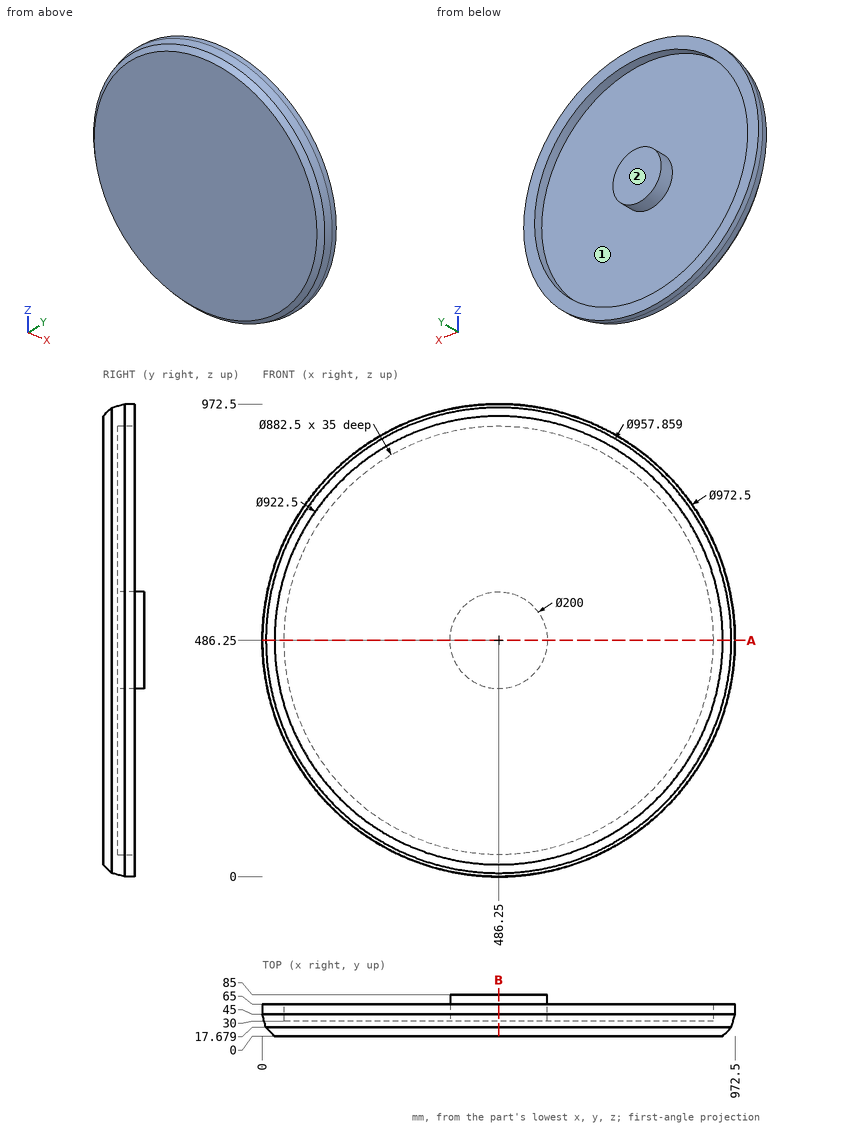
The figure shows three views and two pictorial views of one solid part (mm, origin at its lowest corner). Answer the questions. Give positions to 0.01 mm unless a question says otherwise; leave off trailing zeros. Order: outer loops, then holes, each group sorted by start corner. A loop starts at its lowest first (then second) coordinate and runs counter-clockwise, first axis right, second up. Notation, with made-up numbers: (50, 45.5) -> (75, 45.5) arc R29 ccw to (75, 82.5) -> close; hole circle Ø5 at (-9.75, 75). An arc over 180 degrees is marked (long way). One line per item, written item: value.
1) Find section B-B, the plane x = 486.25. Determine the outline of the cut face in (y, z).
Reported:
outline: (0, 25) -> (17.68, 7.32) -> (45, 0) -> (65, 0) -> (65, 45) -> (30, 45) -> (30, 386.25) -> (85, 386.25) -> (85, 586.25) -> (30, 586.25) -> (30, 927.5) -> (65, 927.5) -> (65, 972.5) -> (45, 972.5) -> (17.68, 965.18) -> (0, 947.5) -> close
2) Find section A-A, the plane z = 486.25. Determine the outline of the cut face in (x, y).
Reported:
outline: (0, 45) -> (7.32, 17.68) -> (25, 0) -> (947.5, 0) -> (965.18, 17.68) -> (972.5, 45) -> (972.5, 65) -> (927.5, 65) -> (927.5, 30) -> (586.25, 30) -> (586.25, 85) -> (386.25, 85) -> (386.25, 30) -> (45, 30) -> (45, 65) -> (0, 65) -> close
3) Find the intervals of material crossed by line 1 (X direction, y = 48, z = 486.25); line 2 (Y direction, x = 440, z = 801.5), in increasing order.
Reported:
line 1: x = 0 to 45, 386.25 to 586.25, 927.5 to 972.5
line 2: y = 0 to 30
4) Determine the mould class of the marked faces 1 and 2 for opening direction X: pulls with the +X half, pulls with the -X half, needs draft (parallel to the pull), parting line crosses it, or undercut.
Reported:
face 1: undercut
face 2: needs draft
5) Flat-ended cylindrical pins translate along their axes: P1, Ø2, axis at y = 48.5, z = 118, coming from the -X side (1 decimal); P2, Ø3, axis at x = 176.5, y = 43, coming from the +Z side; P3, Ø5, axis at y = 61.5, z = 708, coming from the +X side (1 decimal). Find the tip coordinate at first contact, or state that the pin passes through.
Reported:
P1: stops at x = 167.6
P2: stops at z = 861.72
P3: stops at x = 920.3
